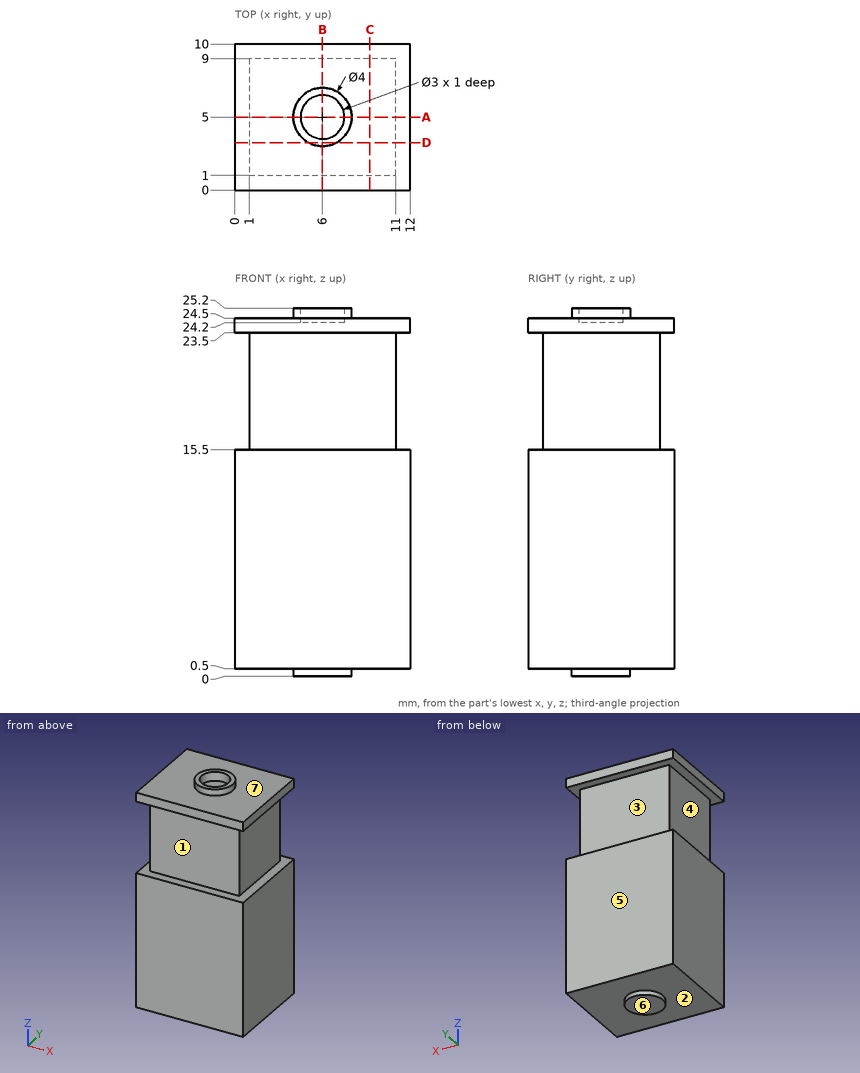
Check sheet for the drawn part. Datum: minimum x, y, z corner. Units: mm. A direction names the side the tool comes from. Round coordinates to 2 decimals unless told otherwise and drop trailing zeros. Order: outer loops, then holes, each group sorted by start corner. A loop starts at its lowest first (then second) coordinate and runs counter-clockwise, first axis right, second up. Notation, with made-up numbers: M 19.5,-28.5 L 65.5,-28.5 A12 cw 65.5,-8.5 Z; hole C 61,36 d3. An arc over 180 degrees is marked long. Answer in a Markdown table with one row per item.
(1) Section check D-D on y = 3.25. Record the boundary of the cut face in (x, z).
Findings:
| item | result |
|---|---|
| outline | M 0,0.5 L 5.03,0.5 L 5.03,0 L 6.97,0 L 6.97,0.5 L 12,0.5 L 12,15.5 L 11,15.5 L 11,23.5 L 12,23.5 L 12,24.5 L 6.97,24.5 L 6.97,25.2 L 5.03,25.2 L 5.03,24.5 L 0,24.5 L 0,23.5 L 1,23.5 L 1,15.5 L 0,15.5 Z |
(2) Draft check along Z on the marked faces 4, 5, 6 and 7. Enter one of: +Z half, -Z half, draft (parallel to the pull), parting line (faces both ways), or undercut.
Findings:
| item | result |
|---|---|
| face 4 | undercut |
| face 5 | draft |
| face 6 | -Z half |
| face 7 | +Z half |
(3) Section check C-C on x = 9.25. Record the boundary of the cut face in (y, z).
Findings:
| item | result |
|---|---|
| outline | M 0,0.5 L 10,0.5 L 10,15.5 L 9,15.5 L 9,23.5 L 10,23.5 L 10,24.5 L 0,24.5 L 0,23.5 L 1,23.5 L 1,15.5 L 0,15.5 Z |
(4) Set-up check for the marked faces 1, 2 and 3: record each of +Z, -Z, +X, -X, +Y, -Y from which the full face is reachable in a straight line by a thin tool's end or side.
Findings:
| item | result |
|---|---|
| face 1 | +X, -X, -Y |
| face 2 | -Z |
| face 3 | +X, -X, +Y |
(5) Material ranges on line 1 along Z through (x, y) = (0.5, 2.25); line 2 along Y through (x, z) = (6, 24.85); line 3 along Z through (x, y) = (5, 5.25), recorded low to high. Write a range as from..to.
Findings:
| item | result |
|---|---|
| line 1 | z = 0.5..15.5, 23.5..24.5 |
| line 2 | y = 3..3.5, 6.5..7 |
| line 3 | z = 0..24.2 |
(6) Section check A-A on y = 5. Record the boundary of the cut face in (x, z).
Findings:
| item | result |
|---|---|
| outline | M 0,0.5 L 4,0.5 L 4,0 L 8,0 L 8,0.5 L 12,0.5 L 12,15.5 L 11,15.5 L 11,23.5 L 12,23.5 L 12,24.5 L 8,24.5 L 8,25.2 L 7.5,25.2 L 7.5,24.2 L 4.5,24.2 L 4.5,25.2 L 4,25.2 L 4,24.5 L 0,24.5 L 0,23.5 L 1,23.5 L 1,15.5 L 0,15.5 Z |
(7) Gauge pin test, flat ends, axial feed: pin 1 (1 mm diameter, centred on y = 6, z = 14, fed in from -X); pin 2 (2.5 mm diameter, centred on y = 6.5, z = 18.5, fed in from -X); pin 3 (4 mm diameter, centred on x = 4.5, z = 18, fed in from -Y); pin 4 (2 mm diameter, centred on x = 5, z = 22, fed in from +Y). Record the tip position at first contact, or that the pin passes through.
Findings:
| item | result |
|---|---|
| pin 1 | stops at x = 0 |
| pin 2 | stops at x = 1 |
| pin 3 | stops at y = 1 |
| pin 4 | stops at y = 9 |
(8) Section check B-B on x = 6. Record the boundary of the cut face in (y, z), plus the area to 3 significant figures.
Findings:
| item | result |
|---|---|
| outline | M 0,0.5 L 3,0.5 L 3,0 L 7,0 L 7,0.5 L 10,0.5 L 10,15.5 L 9,15.5 L 9,23.5 L 10,23.5 L 10,24.5 L 7,24.5 L 7,25.2 L 6.5,25.2 L 6.5,24.2 L 3.5,24.2 L 3.5,25.2 L 3,25.2 L 3,24.5 L 0,24.5 L 0,23.5 L 1,23.5 L 1,15.5 L 0,15.5 Z |
| area | 226 mm^2 |
